Geometry: final body of the model. Coordinates: model frame, mm. Face numbers are marked on the shaded views. A direction names the side the tool comes from. Give positions to 0.01 mm unless a question says otherwise; leave off trailing zeros. Write each loop counter-clockwise with the first axis right and the second up, starting at its lowest first coordinate (ties: lowest second). Pieces come first, ordered by that corner, then holes. Notation, with made-up numbers: (-35, -10) -> (12, -10) arc R20 cw to (12, 3) -> close; hole circle Ø8 at (59.25, 57.5). An arc over 180 degrees is marked (long way). Answer as a JSON object with one key per item and string values. Group by question number.
(1) Set-up query: the marked faces 1 and 2. Return all of +Z, -Z, +X, -X, +Y, -Y with unobstructed straight access to the full face (end or side cutting, diameter ignored); none if empty.
(2) Section query B-B on z = -21. Output: boundary loops of the cut face in (x, y), plus the area to 3 significant figures.
(3) Material intervals for probe 1 along X at (y, z) = (0, -60.45); probe 2 along X at (y, z) = (0.25, -49.5); probe 3 along Z at (x, y) = (-4.5, -1.75), sorted ascending.
(4) Draft query along X for the marked faces 3, 4 and 5. Return one class per face: +X half, -X half, draft (parallel to the pull), parting line (faces both ways), or undercut.
(5) Section query A-A on z = -10. Output: boundary loops of the cut face in (x, y), plus the area to 3 significant figures.
(6) Contact query for flat-ended pins moving along their axis: pin 1 Ø3 at (x, y) = (0, 0) entering from +Z; pin 2 Ø5 at (x, y) = (-0.5, 0) entering from -Z; pin 3 Ø1.5 at (y, z) = (1, -43.5) entering from +X; pin 4 Ø4 at (x, z) = (2.5, -48) entering from +Y. Output: stop coordinate, or through.
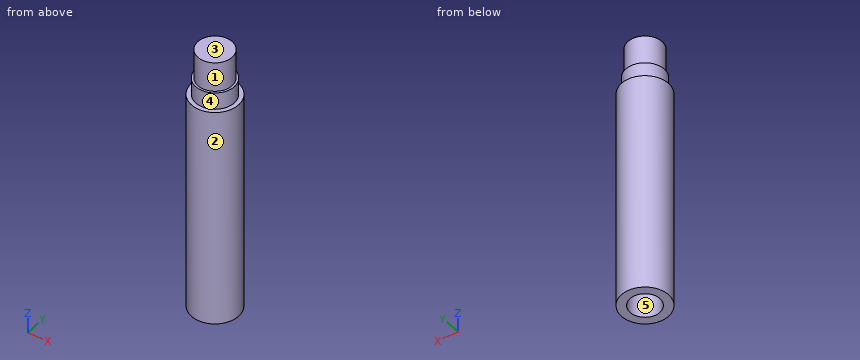
from build123d import *

# Parameters (mm, degrees)
TAP_DRILL_FOR_M8X1_0_TAP1_D     = 7
TAP_DRILL_FOR_M8X1_0_TAP1_DEPTH = 6
TAP_DRILL_FOR_M8X1_0_TAP1_TIP   = 2.103012167


with BuildPart() as part:
    # Sketch1 → Revolve1 (revolve)
    with BuildSketch(Plane(origin=(0, 0, 0), x_dir=(0, 0, -1), z_dir=(1, 0, 0))):
        Polygon((0, 0), (22.670726421, 0), (24, 2.5), (63, 2.5), (63, 5.5), (11, 5.5), (11, 4.5), (7, 4.5), (7, 4), (0, 4), align=None)
    revolve(axis=Axis((0, 0, 0), (0, 0, -1)))

    # Tap Drill for M8x1.0 Tap1
    with Locations(Plane(origin=(0, 0, -63), x_dir=(-1, 0, 0), z_dir=(0, 0, -1))):
        with Locations((0, 0)):
            Hole(TAP_DRILL_FOR_M8X1_0_TAP1_D / 2, depth=TAP_DRILL_FOR_M8X1_0_TAP1_DEPTH)
            with Locations((0, 0, -(TAP_DRILL_FOR_M8X1_0_TAP1_DEPTH + TAP_DRILL_FOR_M8X1_0_TAP1_TIP / 2))):  # 118° drill point
                Cone(0, TAP_DRILL_FOR_M8X1_0_TAP1_D / 2, TAP_DRILL_FOR_M8X1_0_TAP1_TIP, mode=Mode.SUBTRACT)


solid = part.part
Answer list:
{
 "1": {"face 1": "+Z", "face 2": "+Z, -Z"},
 "2": {"outline": "circle Ø11 at (0, 0)", "area": "95.0 mm2"},
 "3": {"probe 1": "-5.5 to -3.5, 3.5 to 5.5", "probe 2": "-5.49 to -2.49, 2.49 to 5.49", "probe 3": "-63 to -11"},
 "4": {"face 3": "draft", "face 4": "parting line", "face 5": "undercut"},
 "5": {"outline": "circle Ø9 at (0, 0)", "area": "63.6 mm2"},
 "6": {"pin 1": "z = 0", "pin 2": "z = -56.7", "pin 3": "x = 5.49", "pin 4": "y = 5.48"}
}
